```python
from build123d import *

# Parameters (mm, degrees)
SKETCH1_R                = 34
BOSS_EXTRUDE1_DEPTH      = 10
SKETCH2_R                = 19.7871926
SKETCH2_R_2              = 2
CUT_EXTRUDE1_DEPTH       = 10
SKETCH3_R                = 4.837531333
SKETCH4_W                = 4.837531333
SKETCH4_H                = 4.837531333
CUT_EXTRUDE3_DEPTH       = 38
CUT_EXTRUDE3_DEPTH_BACK  = 38
SKETCH5_W                = 72.361656805
SKETCH5_H                = 8.896778435
BOSS_EXTRUDE2_START      = 60
SKETCH6_R                = 22.2871926
SKETCH6_R_2              = 19.7871926
BOSS_EXTRUDE2_DEPTH      = 60
SKETCH7_R                = 21.0371926
SKETCH7_R_2              = 19.7871926
CUT_EXTRUDE4_DEPTH       = 25
CUT_EXTRUDE6_DEPTH       = 25
CUT_EXTRUDE6_DEPTH_BACK  = 25
SKETCH8_R                = 2
CUT_EXTRUDE7_DEPTH       = 43
CUT_EXTRUDE7_DEPTH_BACK  = 53
SKETCH9_W                = 69.351432881
SKETCH9_H                = 5.737807944
CUT_EXTRUDE8_START       = -25
SKETCH10_R               = 22.2871926
SKETCH10_R_2             = 21.0371926
CUT_EXTRUDE8_DEPTH       = 25
CUT_EXTRUDE9_DEPTH       = 30
CUT_EXTRUDE9_DEPTH_BACK  = 30
SKETCH11_R               = 2
CUT_EXTRUDE10_DEPTH      = 30
CUT_EXTRUDE10_DEPTH_BACK = 30
SKETCH12_W               = 44.5743852
SKETCH12_H               = 21.576749043
BOSS_EXTRUDE3_DEPTH      = 66
BOSS_EXTRUDE3_DEPTH_BACK = 54
SKETCH13_W               = 10
SKETCH13_H               = 10
CUT_EXTRUDE11_START      = -66
SKETCH14_R               = 19.7871926
CUT_EXTRUDE11_DEPTH      = 66
SKETCH18_W               = 9.329915791
SKETCH18_H               = 10
CUT_EXTRUDE12_DEPTH      = 66
SKETCH19_R               = 2
CUT_EXTRUDE13_DEPTH      = 66
SKETCH20_R               = 58.570053226
SKETCH20_R_2             = 42.40739525
CUT_EXTRUDE14_DEPTH      = 66
SKETCH22_R               = 21.0371926
SKETCH22_R_2             = 19.7871926
BOSS_EXTRUDE4_DEPTH      = 12
CUT_EXTRUDE15_DEPTH      = 66
CUT_EXTRUDE15_DEPTH_BACK = 66
SKETCH21_W               = 15
SKETCH21_H               = 10


with BuildPart() as part:
    # Sketch1 → Boss-Extrude1 (new body)
    with BuildSketch(Plane(origin=(0, 0, 0), x_dir=(1, 0, 0), z_dir=(0, 1, 0))):
        with Locations(Location((0, 0, 0), (0, 0, 270))):
            Circle(SKETCH1_R)
    extrude(amount=BOSS_EXTRUDE1_DEPTH)

    # Sketch2 → Cut-Extrude1 (cut)
    with BuildSketch(Plane.XZ):
        with Locations(Location((0, 0, 0), (0, 0, 270))):
            Circle(SKETCH2_R)
        with Locations(Location((-22.1, 12.5, 0), (0, 0, 270))):
            Circle(SKETCH2_R_2)
        with Locations(Location((22.1, 12.5, 0), (0, 0, 90))):
            Circle(SKETCH2_R_2)
        with Locations(Location((22.1, -12.5, 0), (0, 0, 270))):
            Circle(SKETCH2_R_2)
        with Locations(Location((-22.1, -12.5, 0), (0, 0, 90))):
            Circle(SKETCH2_R_2)
    extrude(amount=-CUT_EXTRUDE1_DEPTH, mode=Mode.SUBTRACT)

    # Sketch3 → Cut-Revolve1 (revolve, cut)
    with BuildSketch(Plane(origin=(0, 0, 0), x_dir=(0, 0, -1), z_dir=(1, 0, 0)), mode=Mode.PRIVATE) as cut_revolve1_sk:
        with Locations((-34, 5)):
            Circle(SKETCH3_R)
    revolve(cut_revolve1_sk.sketch.rotate(Axis((0, 0, 0), (0, 1, 0)), 180), axis=Axis((0, 0, 0), (0, 1, 0)), mode=Mode.SUBTRACT)

    # Sketch4 → Cut-Revolve2 (revolve, cut)
    with BuildSketch(Plane(origin=(0, 0, 0), x_dir=(0, 0, -1), z_dir=(1, 0, 0)), mode=Mode.PRIVATE) as cut_revolve2_sk:
        with Locations((-31.581234333, 2.581234333)):
            Rectangle(SKETCH4_W, SKETCH4_H)
    revolve(cut_revolve2_sk.sketch.rotate(Axis((0, 0, 0), (0, 1, 0)), 180), axis=Axis((0, 0, 0), (0, 1, 0)), mode=Mode.SUBTRACT)

    # Sketch5 → Cut-Extrude3 (cut, two sides: drawn at the far end of the back side and taken through both)
    with BuildSketch(Plane(origin=(0, 0, 0), x_dir=(0, 0, -1), z_dir=(1, 0, 0)).offset(-CUT_EXTRUDE3_DEPTH_BACK)):
        with Locations((-0.901301775, 0.551610782)):
            Rectangle(SKETCH5_W, SKETCH5_H)
    extrude(amount=CUT_EXTRUDE3_DEPTH + CUT_EXTRUDE3_DEPTH_BACK, mode=Mode.SUBTRACT)

    # Sketch6 → Boss-Extrude2 (add)
    with BuildSketch(Plane.XZ.offset(-5).offset(BOSS_EXTRUDE2_START)):
        with Locations(Location((0, 0, 0), (0, 0, 270))):
            Circle(SKETCH6_R)
        with Locations(Location((0, 0, 0), (0, 0, 270))):
            Circle(SKETCH6_R_2, mode=Mode.SUBTRACT)
    extrude(amount=-BOSS_EXTRUDE2_DEPTH)

    # Sketch7 → Cut-Extrude4 (cut)
    with BuildSketch(Plane.XZ.offset(55)):
        with Locations(Location((0, 0, 0), (0, 0, 270))):
            Circle(SKETCH7_R)
        with Locations(Location((0, 0, 0), (0, 0, 270))):
            Circle(SKETCH7_R_2, mode=Mode.SUBTRACT)
    extrude(amount=-CUT_EXTRUDE4_DEPTH, mode=Mode.SUBTRACT)

    # Sketch8 → Cut-Extrude6 (cut, two sides: drawn at the far end of the back side and taken through both)
    with BuildSketch(Plane(origin=(0, 0, 0), x_dir=(0, 0, -1), z_dir=(1, 0, 0)).offset(-CUT_EXTRUDE6_DEPTH_BACK)):
        with Locations(Location((0, -42.5, 0), (0, 0, 180))):
            Circle(SKETCH8_R)
    extrude(amount=CUT_EXTRUDE6_DEPTH + CUT_EXTRUDE6_DEPTH_BACK, mode=Mode.SUBTRACT)

    # Sketch9 → Cut-Extrude7 (cut, two sides: drawn at the far end of the back side and taken through both)
    with BuildSketch(Plane(origin=(0, 0, 0), x_dir=(0, 0, -1), z_dir=(1, 0, 0)).offset(-CUT_EXTRUDE7_DEPTH_BACK)):
        with Locations((0.165912519, 7.868903972)):
            Rectangle(SKETCH9_W, SKETCH9_H)
    extrude(amount=CUT_EXTRUDE7_DEPTH + CUT_EXTRUDE7_DEPTH_BACK, mode=Mode.SUBTRACT)

    # Sketch10 → Cut-Extrude8 (cut)
    with BuildSketch(Plane(origin=(0, 5, 0), x_dir=(1, 0, 0), z_dir=(0, 1, 0)).offset(CUT_EXTRUDE8_START)):
        with Locations(Location((0, 0, 0), (0, 0, 270))):
            Circle(SKETCH10_R)
        with Locations(Location((0, 0, 0), (0, 0, 90))):
            Circle(SKETCH10_R_2, mode=Mode.SUBTRACT)
    extrude(amount=CUT_EXTRUDE8_DEPTH, mode=Mode.SUBTRACT)

    # Sketch11 → Cut-Extrude9 (cut, two sides: drawn at the far end of the back side and taken through both)
    with BuildSketch(Plane(origin=(0, 0, 0), x_dir=(0, 0, -1), z_dir=(1, 0, 0)).offset(-CUT_EXTRUDE9_DEPTH_BACK)):
        with Locations(Location((0, -7.5, 0), (0, 0, 180))):
            Circle(SKETCH11_R)
    extrude(amount=CUT_EXTRUDE9_DEPTH + CUT_EXTRUDE9_DEPTH_BACK, mode=Mode.SUBTRACT)

    # Sketch12 → Cut-Extrude10 (cut, two sides: drawn at the far end of the back side and taken through both)
    with BuildSketch(Plane(origin=(0, 0, 0), x_dir=(0, 0, -1), z_dir=(1, 0, 0)).offset(-CUT_EXTRUDE10_DEPTH_BACK)):
        with Locations((0, -44.211625478)):
            Rectangle(SKETCH12_W, SKETCH12_H)
    extrude(amount=CUT_EXTRUDE10_DEPTH + CUT_EXTRUDE10_DEPTH_BACK, mode=Mode.SUBTRACT)

    # Sketch13 → Boss-Extrude3 (add, two sides: drawn at the far end of the back side and taken through both)
    with BuildSketch(Plane(origin=(0, 0, 0), x_dir=(0, 0, -1), z_dir=(1, 0, 0)).offset(-BOSS_EXTRUDE3_DEPTH_BACK)):
        with Locations((0, -28.423250957)):
            Rectangle(SKETCH13_W, SKETCH13_H)
    extrude(amount=BOSS_EXTRUDE3_DEPTH + BOSS_EXTRUDE3_DEPTH_BACK)

    # Sketch14 → Cut-Extrude11 (cut)
    with BuildSketch(Plane(origin=(0, -23.423250957, 0), x_dir=(1, 0, 0), z_dir=(0, 1, 0)).offset(CUT_EXTRUDE11_START)):
        with Locations(Location((0, 0, 0), (0, 0, 14.636672901))):
            Circle(SKETCH14_R)
    extrude(amount=CUT_EXTRUDE11_DEPTH, mode=Mode.SUBTRACT)

    # Sketch17 → Cut-Revolve5 (revolve, cut)
    with BuildSketch(Plane.XY, mode=Mode.PRIVATE) as cut_revolve5_sk:
        with BuildLine():
            Line((-56.890231537, -28.423250957), (-27.2871926, -28.423250957))
            ThreePointArc((-27.2871926, -28.423250957), (-23.751658694, -19.887717051), (-32.2871926, -23.423250957))
            Line((-32.2871926, -23.423250957), (-56.890231537, -23.423250957))
            Line((-56.890231537, -23.423250957), (-56.890231537, -28.423250957))
        make_face()
    revolve(cut_revolve5_sk.sketch.rotate(Axis((0, -33.423250957, 0), (0, 1, 0)), 90), axis=Axis((0, -33.423250957, 0), (0, 1, 0)), mode=Mode.SUBTRACT)

    # Sketch18 → Cut-Extrude12 (cut)
    with BuildSketch(Plane.XY.offset(5)):
        with Locations((61.335042105, -28.423250957)):
            Rectangle(SKETCH18_W, SKETCH18_H)
    extrude(amount=-CUT_EXTRUDE12_DEPTH, mode=Mode.SUBTRACT)

    # Sketch19 → Cut-Extrude13 (cut)
    with BuildSketch(Plane.XZ.offset(33.423250957)):
        with Locations(Location((-33.75, 0, 0), (0, 0, 270))):
            Circle(SKETCH19_R)
        with Locations(Location((33.75, 0, 0), (0, 0, 270))):
            Circle(SKETCH19_R)
    extrude(amount=-CUT_EXTRUDE13_DEPTH, mode=Mode.SUBTRACT)

    # Sketch20 → Cut-Extrude14 (cut)
    with BuildSketch(Plane.XZ.offset(33.423250957)):
        Circle(SKETCH20_R)
        Circle(SKETCH20_R_2, mode=Mode.SUBTRACT)
    extrude(amount=-CUT_EXTRUDE14_DEPTH, mode=Mode.SUBTRACT)

    # Sketch22 → Boss-Extrude4 (add)
    with BuildSketch(Plane.XZ.offset(33.423250957)):
        with Locations(Location((0, 0, 0), (0, 0, 90))):
            Circle(SKETCH22_R)
        with Locations(Location((0, 0, 0), (0, 0, 270))):
            Circle(SKETCH22_R_2, mode=Mode.SUBTRACT)
    extrude(amount=-BOSS_EXTRUDE4_DEPTH)

    # Sketch21 → Cut-Extrude15 (cut, two sides: drawn at the far end of the back side and taken through both)
    with BuildSketch(Plane(origin=(0, 0, -5), x_dir=(-1, 0, 0), z_dir=(0, 0, -1)).offset(-CUT_EXTRUDE15_DEPTH_BACK)):
        with Locations((0, -28.423250957)):
            Rectangle(SKETCH21_W, SKETCH21_H)
    extrude(amount=CUT_EXTRUDE15_DEPTH + CUT_EXTRUDE15_DEPTH_BACK, mode=Mode.SUBTRACT)


solid = part.part
```
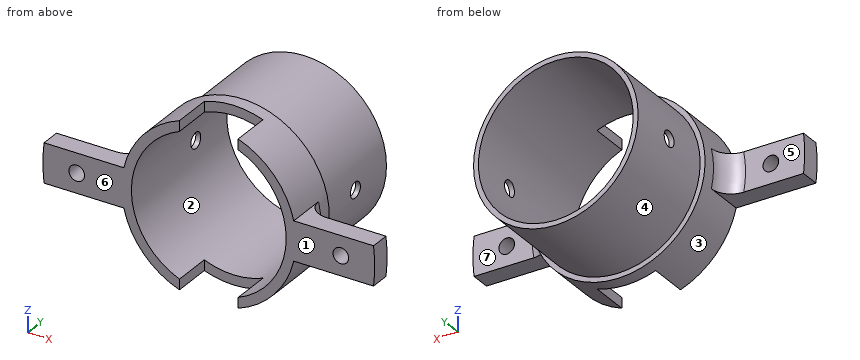
Part model, mm, in its own coordinate system. Face numbers are marked on the shaded views. A direction names the side the tool comes from. Round coordinates to 2 decimals unless told otherwise and drop trailing zeros. Write each loop counter-clockwise with the first axis right and the second up, starting at its lowest first coordinate (ties: lowest second). Pieces come first, ordered by that corner, then holes. Notation, with made-up numbers: (-36, -33.75) -> (-10, -33.75) arc R15 ccw to (-10, -13.75) -> close; hole circle Ø11 at (82, -11). An arc over 180 degrees is marked (long way). Return JSON: item names as keys, results as strings. Group by question number.
Q1. Saw through at B-B on x = 33.75. Write the cut outline in (y, z).
Q2. Mould opens along Z. For the marked faces 1, 2 and 3 say: pulls with the +Z half, pulls with the -Z half, needs draft (parallel to the pull), parting line crosses it, or undercut.
Q3. Probe L1, parallel to Y at x = 20, z = 0; L2, parallel to X at y = -21.5, z = 0; L3, parallel to X at y = -3.5, z = 0. List the from-to ranges inside material, lowest first. Write a range as [from, to].
Q4. Saw through at A-A on z = 0. State how many separate pieces and enclosed holes the cut face has, plus the area to 3 significant figures.
Q5. Saw through at D-D on z = 11.5. Write the cut outline in (x, y).
Q6. Which spindle directions (+Z, -Z, +X, -X, +Y, -Y) get a long thin tool onto all of the face, cutting with end or side? Do the marked faces 4, 5, 6 and 7. Say none if no direction does.
Q7. Pin check, flat tips, straight feed: pin 1 (8 mm diameter, centred on x = 32.5, z = 0.5, fed in from +Y); pin 2 (8 mm diameter, centred on x = -33.5, y = -28.5, fed in from +Z); pin 3 (1.3 mm diameter, centred on y = -26.5, z = 19.5, fed in from +X); pin 4 (1.5 mm diameter, centred on x = 19, z = 4.5, fed in from +Y). Stop position of each tip, or through.
Answer:
{
 "1": {"outline": "(-33.42, -5) -> (-28.42, -5) -> (-28.42, -2) -> (-33.42, -2) -> close; (-33.42, 2) -> (-28.42, 2) -> (-28.42, 5) -> (-33.42, 5) -> close"},
 "2": {"face 1": "needs draft", "face 2": "undercut", "face 3": "parting line crosses it"},
 "3": {"L1": "[-33.42, -9.5], [-5.5, 5]", "L2": "[-22.29, -19.79], [19.79, 22.29]", "L3": "[-21.04, -19.79], [19.79, 21.04]"},
 "4": {"separate pieces": "6", "enclosed holes": "0", "area": "292 mm2"},
 "5": {"outline": "(-19.09, -33.42) -> (-16.1, -33.42) -> (-16.1, 5) -> (-17.62, 5) -> (-17.62, -20) -> (-19.09, -20) -> close; (16.1, -33.42) -> (19.09, -33.42) -> (19.09, -20) -> (17.62, -20) -> (17.62, 5) -> (16.1, 5) -> close"},
 "6": {"face 4": "+Y", "face 5": "+Z, -Z, -X, +Y", "face 6": "+Z, -Z, +X, -X, -Y", "face 7": "+Z, -Z, +X, +Y"},
 "7": {"pin 1": "y = -28.42", "pin 2": "z = 5", "pin 3": "x = 11.89", "pin 4": "y = 5"}
}
